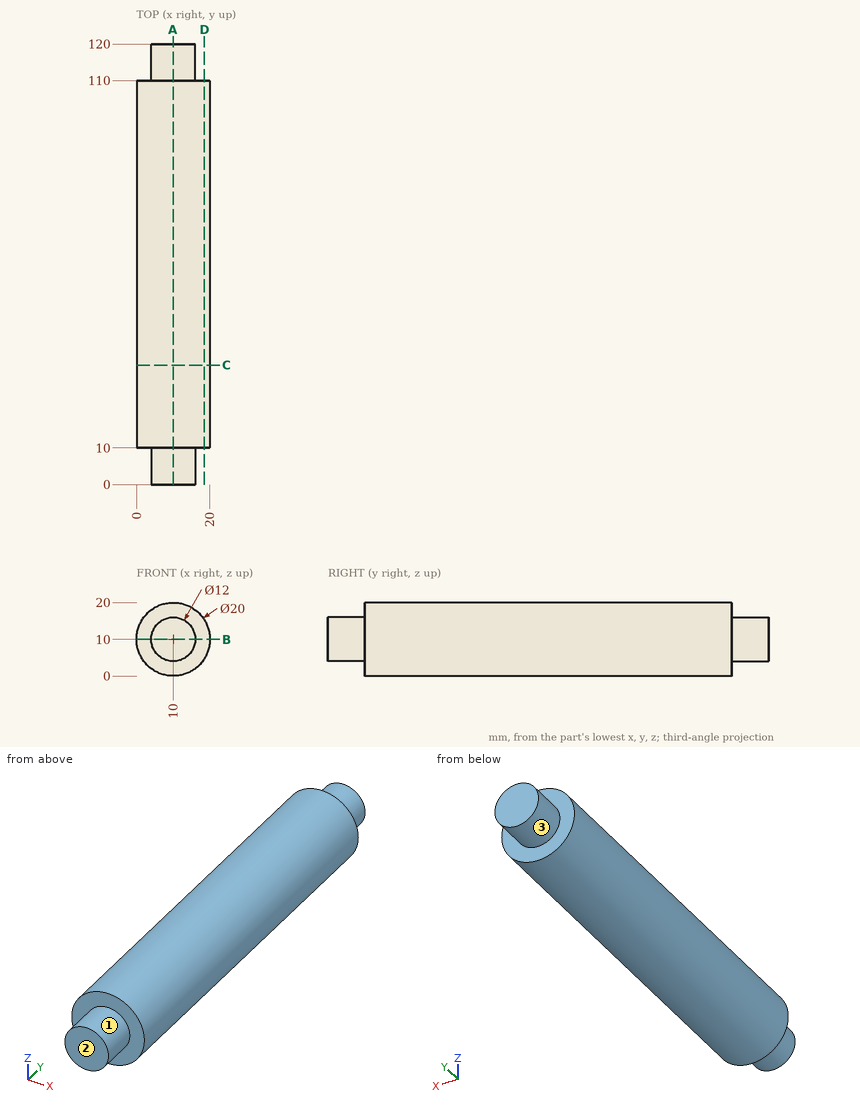
Input: dimensioned drawing with shaded views. Units: mm. Origin: part minimum x, y, z. A direction names the side the tool comes from. Round coordinates to 2 decimals unless told otherwise and drop trailing zeros. Order: outer loops, then holes, each group sorted by start corner. A loop starts at its lowest first (then second) coordinate and runs counter-clockwise, first axis right, second up. Notation, with made-up numbers: (56.25, 85.25) -> (66.25, 85.25) arc R21 cw to (66.25, 109.25) -> close; hole circle Ø1 at (-37.75, -35.75). An arc over 180 degrees is marked (long way). One line per item, written item: value. Start each with the question number.
Q1. Section query D-D (x = 18.5). Return the cut outline in (y, z).
Q2. Access query for the marked faces 1, 2 and 3. Directions: +Z, -Z, +X, -X, +Y, -Y. A direction counts if a zero-diameter tool reaches every point of the face in a straight line with its end or side. Return the directions, or none.
Q3. Material intervals for probe 1 along Y at (x, z) = (4.75, 5.25); probe 2 along Z at (x, y) = (10.5, 50.5); probe 3 along Z at (x, y) = (1, 100), sorted ascending.
Q4. Section query A-A (x = 10). Return the cut outline in (y, z), plus the area to 3 significant figures.
Q5. Section query B-B (z = 10). Return the cut outline in (x, y), plus the area to 3 significant figures.
Q6. Pin query (flat end, axial travel): pin 1 (4 mm diameter, centred on y = 41.5, z = 11.5, fed in from -X); pin 2 (1.5 mm diameter, centred on y = 24, z = 16, fed in from +X). Return the tip coordinate at first contact, or that it passes through.
Q7. Section query C-C (y = 32.5). Return the cut outline in (x, z).
Findings below:
1. outline: (10, 4.73) -> (110, 4.73) -> (110, 15.27) -> (10, 15.27) -> close
2. face 1: -Y
2. face 2: +Z, -Z, +X, -X, -Y
2. face 3: +Y
3. probe 1: 10 to 110
3. probe 2: 0.01 to 19.99
3. probe 3: 5.64 to 14.36
4. outline: (0, 4) -> (10, 4) -> (10, 0) -> (110, 0) -> (110, 4) -> (120, 4) -> (120, 16) -> (110, 16) -> (110, 20) -> (10, 20) -> (10, 16) -> (0, 16) -> close
4. area: 2,240 mm²
5. outline: (0, 10) -> (4, 10) -> (4, 0) -> (16, 0) -> (16, 10) -> (20, 10) -> (20, 110) -> (16, 110) -> (16, 120) -> (4, 120) -> (4, 110) -> (0, 110) -> close
5. area: 2,240 mm²
6. pin 1: x = 0
6. pin 2: x = 18.51
7. outline: circle Ø20 at (10, 10)
